from build123d import *

# Parameters (mm, degrees)
BASE_EXTRUDE_DEPTH  = 25.4
SKETCH7_W           = 12.7
SKETCH7_H           = 38.1
BOSS_EXTRUDE5_DEPTH = 25.4
SKETCH8_W           = 25.751736715
SKETCH8_H           = 25.4
CUT_EXTRUDE5_DEPTH  = 25.4
SKETCH11_W          = 12.7
SKETCH11_H          = 38.1
BOSS_EXTRUDE6_DEPTH = 25.4
SKETCH12_W          = 25.4
SKETCH12_H          = 25.4
CUT_EXTRUDE7_DEPTH  = 20.32
SKETCH13_R          = 7.62
CUT_EXTRUDE8_DEPTH  = 20.32
SKETCH14_R          = 7.62
CUT_EXTRUDE9_DEPTH  = 50.8


with BuildPart() as part:
    # Sketch1 → Base-Extrude (new body)
    with BuildSketch(Plane.XY):
        Polygon((-4.57611336, -135.706612686), (-29.97611336, -135.706612686), (-29.97611336, 29.393387314), (-55.37611336, 29.393387314), (-55.37611336, 67.493387314), (-29.97611336, 67.493387314), (-4.57611336, 67.493387314), align=None)
    extrude(amount=-BASE_EXTRUDE_DEPTH)

    # Sketch7 → Boss-Extrude5 (add)
    with BuildSketch(Plane.ZY.offset(29.97611336)):
        with Locations((-31.75, -116.656612686)):
            Rectangle(SKETCH7_W, SKETCH7_H)
        with Locations((6.35, -116.656612686)):
            Rectangle(SKETCH7_W, SKETCH7_H)
    extrude(amount=-BOSS_EXTRUDE5_DEPTH)

    # Sketch8 → Cut-Extrude5 (cut)
    with BuildSketch(Plane.ZY.offset(29.97611336)):
        with Locations((-12.524131643, -123.006612686)):
            Rectangle(SKETCH8_W, SKETCH8_H)
    extrude(amount=-CUT_EXTRUDE5_DEPTH, mode=Mode.SUBTRACT)

    # Sketch11 → Boss-Extrude6 (add)
    with BuildSketch(Plane(origin=(-4.57611336, 0, 0), x_dir=(0, 0, -1), z_dir=(1, 0, 0))):
        with Locations((31.75, 48.443387314)):
            Rectangle(SKETCH11_W, SKETCH11_H)
        with Locations((-6.35, 48.443387314)):
            Rectangle(SKETCH11_W, SKETCH11_H)
    extrude(amount=-BOSS_EXTRUDE6_DEPTH)

    # Sketch12 → Cut-Extrude7 (cut)
    with BuildSketch(Plane(origin=(-4.57611336, 0, 0), x_dir=(0, 0, -1), z_dir=(1, 0, 0))):
        with Locations((12.7, 54.793387314)):
            Rectangle(SKETCH12_W, SKETCH12_H)
    extrude(amount=-CUT_EXTRUDE7_DEPTH, mode=Mode.SUBTRACT)

    # Sketch13 → Cut-Extrude8 (cut)
    with BuildSketch(Plane.ZY.offset(55.37611336)):
        with Locations(Location((-13.088541232, 49.429752215, 0), (0, 0, 270))):
            Circle(SKETCH13_R)
    extrude(amount=-CUT_EXTRUDE8_DEPTH, mode=Mode.SUBTRACT)

    # Sketch14 → Cut-Extrude9 (cut)
    with BuildSketch(Plane(origin=(0, 0, -38.1), x_dir=(-1, 0, 0), z_dir=(0, 0, -1))):
        with Locations(Location((16.00611336, 54.793387314, 0), (0, 0, 90))):
            Circle(SKETCH14_R)
        with Locations(Location((17.931310165, -123.006612686, 0), (0, 0, 90))):
            Circle(SKETCH14_R)
    extrude(amount=-CUT_EXTRUDE9_DEPTH, mode=Mode.SUBTRACT)


solid = part.part
Work out the finished part from the listing and answer in its coordinate system (mm). A direction names the side the tool comes from. Give positions to 0.01 mm unless a question says otherwise; leave off trailing zeros. Order: outer loops, then holes, each group sorted by start corner. A loop starts at its lowest first (then second) coordinate and runs counter-clockwise, first axis right, second up. Notation, with made-up numbers: (-32.5, 11) -> (6.5, 11) arc R22 ccw to (6.5, 17) -> close; hole circle Ø6 at (-21.5, -9). An arc over 180 degrees is marked (long way). One line per item, written item: value.
Item 1: Find section B-B, the plane y = 51.5. Give the vertices of the cut face in (x, z), plus the area to 3 significant figures.
Answer sheet:
outline: (-55.38, -25.4) -> (-29.98, -25.4) -> (-29.98, -38.1) -> (-22.88, -38.1) -> (-22.88, -25.4) -> (-24.9, -25.4) -> (-24.9, 0) -> (-22.88, 0) -> (-22.88, 12.7) -> (-29.98, 12.7) -> (-29.98, 0) -> (-55.38, 0) -> (-55.38, -5.76) -> (-35.06, -5.76) -> (-35.06, -20.42) -> (-55.38, -20.42) -> close; (-9.13, -38.1) -> (-4.58, -38.1) -> (-4.58, -25.4) -> (-9.13, -25.4) -> close; (-9.13, 0) -> (-4.58, 0) -> (-4.58, 12.7) -> (-9.13, 12.7) -> close
area: 772 mm²
Item 2: Find section D-D, the plane y = -20. Give the vertices of the cut face in (x, z), plus the area to 3 significant figures.
Answer sheet:
outline: (-29.98, -25.4) -> (-4.58, -25.4) -> (-4.58, 0) -> (-29.98, 0) -> close
area: 645 mm²
Item 3: Find section C-C, the plane z = -3.5. Give the vertices of the cut face in (x, y).
Answer sheet:
outline: (-55.38, 29.39) -> (-29.98, 29.39) -> (-29.98, -110.31) -> (-4.58, -110.31) -> (-4.58, 42.09) -> (-24.9, 42.09) -> (-24.9, 67.49) -> (-55.38, 67.49) -> close
Item 4: Determine the mould class of faces 1 (the flat face through (-17, 44, 12.7)), 2 (the flat face through (-12, -129, -25.4)), 3 (the flat face through (-42, 29.393, -13)), 4 (the flat face through (-8, 55, 0)) for opening direction Z: released by +Z, released by -Z, zero draft, split by the parting line, or undercut.
Answer sheet:
face 1: released by +Z
face 2: undercut
face 3: zero draft
face 4: undercut
Item 5: Flat-ended cylindrical pins translate along their axes: P1, Ø7.5, axis at x = -22, z = -14.5, coming from the -Y side; P2, Ø20.5, axis at x = -16, y = -53, coming from the +Z side; P3, Ø10, axis at y = 43, z = -34, coming from the -X side. Find the tip coordinate at first contact, or state that the pin passes through.
Answer sheet:
P1: y = -110.31
P2: z = 0
P3: x = -29.98
Item 6: Straight lines are drawn through the part: probe 1 along X at (y, z) = (-19.5, -7.5); probe 2 along Y at (x, z) = (-31, -9); probe 3 along Y at (x, z) = (-14.5, 6). For each, find the intervals that lie inside material, in ascending order.
Answer sheet:
probe 1: -29.98 to -4.58
probe 2: 29.39 to 67.49
probe 3: -135.71 to -129.81, -116.2 to -97.61, 29.39 to 47.32, 62.26 to 67.49
Item 7: A tool of negligible diameter and unlimited length cuts with its end or side. For faces 5 (the flat face through (-8, 55, -25.4)), 6 (the flat face through (-42, 49, -25.4)), 7 (the flat face through (-17, -97.607, -32)), 8 (the flat face through (-29.976, 49, 6)), 9 (the flat face through (-29.976, -52, -13)), from which of +Z, -Z, +X, -X, +Y, -Y can it reach the whole face along a straight path? Write none if from no direction.
Answer sheet:
face 5: +X, +Y
face 6: -Z, -X, +Y, -Y
face 7: -Z, +X, -X
face 8: +Z, -X, +Y, -Y
face 9: +Z, -Z, -X, -Y
Item 8: Find section A-A, the plane z = -34. Give the vertices of the cut face in (x, y).
Answer sheet:
outline: (-29.98, -135.71) -> (-4.58, -135.71) -> (-4.58, -97.61) -> (-29.98, -97.61) -> close; (-29.98, 29.39) -> (-4.58, 29.39) -> (-4.58, 67.49) -> (-29.98, 67.49) -> close; hole circle Ø15.24 at (-17.93, -123.01); hole circle Ø15.24 at (-16.01, 54.79)
